from build123d import *

# Parameters (mm, degrees)
SKETCH1_W           = 168.379590863
SKETCH1_H           = 126.39
BOSS_EXTRUDE1_DEPTH = 70
SKETCH2_W           = 168.379590863
SKETCH2_H           = 126.39
BOSS_EXTRUDE2_DEPTH = 4
SKETCH3_W           = 142.779590863
SKETCH3_H           = 96.34
CUT_EXTRUDE1_DEPTH  = 4
FILLET1_R           = 5
FILLET4_R           = 2
FILLET5_R           = 2
SKETCH4_W           = 10
SKETCH4_H           = 10
CUT_EXTRUDE2_DEPTH  = 195
SKETCH6_R           = 2
CUT_EXTRUDE3_DEPTH  = 195
SKETCH8_R           = 2
CUT_EXTRUDE4_DEPTH  = 195
SKETCH9_W           = 103.95032351
SKETCH9_H           = 88.010158037
CUT_EXTRUDE5_DEPTH  = 201
SKETCH10_W          = 5
SKETCH10_H          = 2
SKETCH10_W_2        = 2
CUT_EXTRUDE6_DEPTH  = 15
SKETCH11_W          = 1.5
SKETCH11_H          = 5
CUT_EXTRUDE7_DEPTH  = 15
SKETCH12_W          = 1.5
SKETCH12_H          = 5
CUT_EXTRUDE8_DEPTH  = 15


with BuildPart() as part:
    # Sketch1 → Boss-Extrude1 (new body)
    with BuildSketch(Plane(origin=(0, 0, 0), x_dir=(1, 0, 0), z_dir=(0, 1, 0))):
        with Locations((4.455204569, -8.048213198)):
            Rectangle(SKETCH1_W, SKETCH1_H)
        Polygon((-76.734590863, 32.146786802), (-76.734590863, 52.146786802), (85.645, 52.146786802), (85.645, -68.243213198), (60.555409137, -68.243213198), (-76.734590863, -68.243213198), align=None, mode=Mode.SUBTRACT)
    extrude(amount=BOSS_EXTRUDE1_DEPTH)

    # Sketch2 → Boss-Extrude2 (add)
    with BuildSketch(Plane(origin=(0, 0, 0), x_dir=(-1, 0, 0), z_dir=(0, -1, 0))):
        with Locations((-4.455204569, -8.048213198)):
            Rectangle(SKETCH2_W, SKETCH2_H)
    extrude(amount=BOSS_EXTRUDE2_DEPTH)

    # Sketch3 → Cut-Extrude1 (cut)
    with BuildSketch(Plane(origin=(0, 0, 0), x_dir=(1, 0, 0), z_dir=(0, 1, 0))):
        with Locations((9.755204569, 0.476786802)):
            Rectangle(SKETCH3_W, SKETCH3_H)
    extrude(amount=-CUT_EXTRUDE1_DEPTH, mode=Mode.SUBTRACT)

    # Fillet1
    fillet1_edges = [part.edges().sort_by_distance(p)[0] for p in [
        (-79.734590863, 33, -55.146786802),
        (88.645, 33, -55.146786802),
        (88.645, 33, 71.243213198),
        (-79.734590863, 33, 71.243213198),
    ]]
    fillet(fillet1_edges, radius=FILLET1_R)

    # Fillet4
    fillet4_edges = [part.edges().sort_by_distance(p)[0] for p in [
        (4.455204569, -4, 71.243213198),
        (-79.734590863, -4, 8.048213198),
        (4.455204569, -4, -55.146786802),
        (88.645, -4, 8.048213198),
        (87.180533906, -4, 69.778747104),
        (87.180533906, -4, -53.682320708),
        (-78.270124769, -4, -53.682320708),
        (-78.270124769, -4, 69.778747104),
    ]]
    fillet(fillet4_edges, radius=FILLET4_R)

    # Fillet5
    fillet5_edges = [part.edges().sort_by_distance(p)[0] for p in [
        (81.145, -4, -0.476786802),
        (9.755204569, -4, 47.693213198),
        (-61.634590863, -4, -0.476786802),
        (9.755204569, -4, -48.646786802),
    ]]
    fillet(fillet5_edges, radius=FILLET5_R)

    # Sketch4 → Cut-Extrude2 (cut)
    with BuildSketch(Plane.ZY.offset(79.734590863)):
        with Locations((5.00870497, 36.749697215)):
            Rectangle(SKETCH4_W, SKETCH4_H)
    extrude(amount=-CUT_EXTRUDE2_DEPTH, mode=Mode.SUBTRACT)

    # Sketch6 → Cut-Extrude3 (cut)
    with BuildSketch(Plane(origin=(88.645, 0, 0), x_dir=(0, 0, -1), z_dir=(1, 0, 0))):
        with Locations((-7.57558331, 65)):
            Circle(SKETCH6_R)
    extrude(amount=-CUT_EXTRUDE3_DEPTH, mode=Mode.SUBTRACT)

    # Sketch8 → Cut-Extrude4 (cut)
    with BuildSketch(Plane(origin=(0, 0, -55.146786802), x_dir=(-1, 0, 0), z_dir=(0, 0, -1))):
        with Locations((-43.645, 65)):
            Circle(SKETCH8_R)
        with Locations((34.734590863, 65)):
            Circle(SKETCH8_R)
    extrude(amount=-CUT_EXTRUDE4_DEPTH, mode=Mode.SUBTRACT)

    # Sketch9 → Cut-Extrude5 (cut)
    with BuildSketch(Plane.XY.offset(71.243213198)):
        with Locations((-47.519957186, 25.994920982)):
            Rectangle(SKETCH9_W, SKETCH9_H)
    extrude(amount=-CUT_EXTRUDE5_DEPTH, mode=Mode.SUBTRACT)

    # Sketch10 → Cut-Extrude6 (cut)
    with BuildSketch(Plane.ZY.offset(-4.455204569)):
        with Locations((55.193213198, -1)):
            Rectangle(SKETCH10_W, SKETCH10_H)
        with Locations((65.193213198, -1)):
            Rectangle(SKETCH10_W, SKETCH10_H)
        with Locations((-51.146786802, -1)):
            Rectangle(SKETCH10_W_2, SKETCH10_H)
    extrude(amount=-CUT_EXTRUDE6_DEPTH, mode=Mode.SUBTRACT)

    # Sketch11 → Cut-Extrude7 (cut)
    with BuildSketch(Plane.ZY.offset(-4.455204569)):
        with Locations((68.993213198, 62.5)):
            Rectangle(SKETCH11_W, SKETCH11_H)
        with Locations((68.993213198, 52.5)):
            Rectangle(SKETCH11_W, SKETCH11_H)
        with Locations((68.993213198, 42.5)):
            Rectangle(SKETCH11_W, SKETCH11_H)
        with Locations((68.993213198, 32.5)):
            Rectangle(SKETCH11_W, SKETCH11_H)
        with Locations((68.993213198, 22.5)):
            Rectangle(SKETCH11_W, SKETCH11_H)
        with Locations((68.993213198, 12.5)):
            Rectangle(SKETCH11_W, SKETCH11_H)
    extrude(amount=-CUT_EXTRUDE7_DEPTH, mode=Mode.SUBTRACT)

    # Sketch12 → Cut-Extrude8 (cut)
    with BuildSketch(Plane.ZY.offset(-4.455204569)):
        with Locations((-52.896786802, 57.5)):
            Rectangle(SKETCH12_W, SKETCH12_H)
        with Locations((-52.896786802, 67.5)):
            Rectangle(SKETCH12_W, SKETCH12_H)
        with Locations((-52.896786802, 47.5)):
            Rectangle(SKETCH12_W, SKETCH12_H)
        with Locations((-52.896786802, 37.5)):
            Rectangle(SKETCH12_W, SKETCH12_H)
        with Locations((-52.896786802, 27.5)):
            Rectangle(SKETCH12_W, SKETCH12_H)
        with Locations((-52.896786802, 17.5)):
            Rectangle(SKETCH12_W, SKETCH12_H)
    extrude(amount=-CUT_EXTRUDE8_DEPTH, mode=Mode.SUBTRACT)


solid = part.part
Geometry: final body of the model. Coordinates: model frame, mm. A direction names the side the tool comes from. Round coordinates to 2 decimals unless told otherwise and drop trailing zeros. Write each loop counter-clockwise with the first axis right and the second up, starting at its lowest first coordinate (ties: lowest second). Pieces come first, ordered by that corner, then holes. Notation, with made-up numbers: M 72,72.5 L 125,72.5 A21 cw 125,80.5 Z; hole C 67,77 d6. An arc over 180 degrees is marked long. Write item = value, one per line.
Item 1: Material intervals for line 1 along Z through (x, y) = (33.5, 0.5); line 2 along X through (y, z) = (50.5, -9) (3 decimals); line 3 along Y through (x, z) = (84.5, 33.5), sorted ascending. Write a range as [from, to].
Findings:
line_1 = [-55.15, -52.15], [68.24, 71.24]
line_2 = [85.645, 88.645]
line_3 = [-4, 0]
Item 2: Pin query (flat end, axial travel): P1, Ø1.6, axis at y = -0.5, z = -51, coming from the -X side; P2, Ø1.2, axis at y = 22, z = 69.5, coming from the -X side; P3, Ø0.9, axis at x = 86.5, y = 36.5, coming from the +Z side. Return the tip coordinate at first contact, or that it passes through.
Findings:
P1 = 19.46
P2 = 4.46
P3 = 70.63
Item 3: Section query C-C on y = 52. Return loops of the section in (x, z) (3 decimals).
Findings:
outline = M 4.455,-55.147 L 83.645,-55.147 A5 ccw 88.645,-50.147 L 88.645,66.243 A5 ccw 83.645,71.243 L 4.455,71.243 L 4.455,69.743 L 19.455,69.743 L 19.455,68.243 L 85.645,68.243 L 85.645,-52.147 L 4.455,-52.147 Z
Item 4: Section query D-D on y = 5. Return loops of the section in (x, z) (3 decimals).
Findings:
outline = M 4.455,-55.147 L 83.645,-55.147 A5 ccw 88.645,-50.147 L 88.645,66.243 A5 ccw 83.645,71.243 L 4.455,71.243 L 4.455,68.243 L 85.645,68.243 L 85.645,-52.147 L 4.455,-52.147 Z
Item 5: Access query for faces 4 (the face through (87, 70, 12)), 5 (the face through (63, 0, 48)), 6 (the face through (45, 35, -55.147)), 7 (the face through (12, 57, -53.647)), 8 (the face through (87, 31.75, 5)). Directions: +Z, -Z, +X, -X, +Y, -Y. A direction counts if a zero-diameter tool reaches every point of the face in a straight line with its end or side. Return the directions, or none.
Findings:
face_4 = +Z, -Z, +X, -X, +Y
face_5 = -X, +Y
face_6 = -Z, +X, -X, +Y, -Y
face_7 = -X
face_8 = +X, -X
Item 6: Section query A-A on x = 69.5. Return loops of the section in (y, z), then the cut area to 3 significant figures.
Findings:
outline = M -4,-53.15 A2 ccw -2,-55.15 L 70,-55.15 L 70,-52.15 L 0,-52.15 L 0,-48.65 L -2,-48.65 A2 ccw -4,-50.65 Z; M -4,49.69 A2 ccw -2,47.69 L 0,47.69 L 0,68.24 L 70,68.24 L 70,71.24 L -2,71.24 A2 ccw -4,69.24 Z
area = 537 mm^2
Item 7: Pull-direction query (Z, two-part tool) for faces 1 (the face through (87.22, 34.5, -53.64)), 2 (the face through (42.57, 66.686, -53.668)), 3 (the face through (44, 33, -52.147)); classes: pulls with the +Z half, pulls with the -Z half, needs draft (parallel to the pull), parting line crosses it, or undercut.
Findings:
face_1 = pulls with the -Z half
face_2 = needs draft
face_3 = undercut
Item 8: Section query B-B on z = -17. Return loops of the section in (x, y) (3 decimals), then the cut area to 3 significant figures.
Findings:
outline = M 81.145,-2 A2 ccw 83.145,-4 L 86.645,-4 A2 ccw 88.645,-2 L 88.645,70 L 85.645,70 L 85.645,0 L 81.145,0 Z
area = 238 mm^2
